```python
from build123d import *

# Parameters (mm, degrees)
F0_W      = 20
F0_H      = 20
F1_DEPTH  = 5
F2_W      = 1.8
F2_H      = 9.1
F2_H_2    = 1.8
F2_W_2    = 9.1
F3_DEPTH  = 2
F4_W      = 9
F4_H      = 1.7
F5_DEPTH  = 4
F6_W      = 9
F6_H      = 1.7
F7_DEPTH  = 4
F8_W      = 10
F8_H      = 2.2
F9_DEPTH  = 4
F10_W     = 10
F10_H     = 2.2
F11_DEPTH = 4
F12_W     = 2
F12_H     = 10
F13_DEPTH = 2.2
F14_W     = 10
F14_H     = 2
F15_DEPTH = 2.2
F16_W     = 9
F16_H     = 1.7
F17_DEPTH = 1.8
F18_W     = 1.7
F18_H     = 9
F19_DEPTH = 1.8


with BuildPart() as f1:
    # F0 (on Top) → F1 (new body)
    with BuildSketch(Plane.XY):
        with Locations((-15.7790486701, 11.8990262393)):
            Rectangle(F0_W, F0_H)
    extrude(amount=F1_DEPTH)

    # F2 (on face) → F3 (join)
    with BuildSketch(Plane.XY.offset(5)):
        with Locations((-15.7790486701, 17.3490262393)):
            Rectangle(F2_W, F2_H)
        with Locations((-15.7790486701, 11.8990262393)):
            Rectangle(F2_W, F2_H_2)
        with Locations((-21.2290486701, 11.8990262393)):
            Rectangle(F2_W_2, F2_H_2)
        with Locations((-10.3290486701, 11.8990262393)):
            Rectangle(F2_W_2, F2_H_2)
        with Locations((-15.7790486701, 6.4490262393)):
            Rectangle(F2_W, F2_H)
    extrude(amount=F3_DEPTH)

    # F4 (on face) → F5 (join)
    with BuildSketch(Plane.XZ.offset(-1.8990262393)):
        with Locations((-15.7790486701, 0.85)):
            Rectangle(F4_W, F4_H)
    extrude(amount=F5_DEPTH)

    # F6 (on face) → F7 (join)
    with BuildSketch(Plane(origin=(-25.7790486701, 0, 0), x_dir=(0, -1, 0), z_dir=(-1, 0, 0))):
        with Locations((-11.8990262393, 0.85)):
            Rectangle(F6_W, F6_H)
    extrude(amount=F7_DEPTH)

    # F8 (on face) → F9 (cut)
    with BuildSketch(Plane(origin=(0, 21.8990262393, 0), x_dir=(-1, 0, 0), z_dir=(0, 1, 0))):
        with Locations((15.7790486701, 1.1)):
            Rectangle(F8_W, F8_H)
    extrude(amount=-F9_DEPTH, mode=Mode.SUBTRACT)

    # F10 (on face) → F11 (cut)
    with BuildSketch(Plane.YZ.offset(-5.7790486701)):
        with Locations((11.8990262393, 1.1)):
            Rectangle(F10_W, F10_H)
    extrude(amount=-F11_DEPTH, mode=Mode.SUBTRACT)

    # F12 (on face) → F13 (cut)
    with BuildSketch(Plane(origin=(0, 0, 2.2), x_dir=(1, 0, 0), z_dir=(0, 0, -1))):
        with Locations((-8.7790486701, -11.8990262393)):
            Rectangle(F12_W, F12_H)
    extrude(amount=-F13_DEPTH, mode=Mode.SUBTRACT)

    # F14 (on face) → F15 (cut)
    with BuildSketch(Plane(origin=(0, 0, 2.2), x_dir=(1, 0, 0), z_dir=(0, 0, -1))):
        with Locations((-15.7790486701, -18.8990262393)):
            Rectangle(F14_W, F14_H)
    extrude(amount=-F15_DEPTH, mode=Mode.SUBTRACT)

    # F16 (on face) → F17 (join)
    with BuildSketch(Plane.XY.offset(1.7)):
        with Locations((-15.7790486701, -1.2509737607)):
            Rectangle(F16_W, F16_H)
    extrude(amount=F17_DEPTH)

    # F18 (on face) → F19 (join)
    with BuildSketch(Plane.XY.offset(1.7)):
        with Locations((-28.9290486701, 11.8990262393)):
            Rectangle(F18_W, F18_H)
    extrude(amount=F19_DEPTH)


solid = f1.part
```
Here's how the part is built. I have some questions about the finished solid (model axes, mm). A direction names the side the tool comes from. Coordinates: 2 decimals unless noted, no trailing zeros. Order: outer loops, then holes, each group sorted by start corner. A loop starts at its lowest first (then second) coordinate and runs counter-clockwise, first axis right, second up.
Item 1: Thinking about a two-plate mould opening in Y: for faces 1 (the face through (-5.779, 12, 3)), 2 (the face through (-16, 19, 4.4)), 3 (the face through (-28, 16.399, 1)), which applies, pulls with the +Y half, pulls with the -Y half, needs draft (parallel to the pull), parting line crosses it, or undercut?
Response values:
face 1: needs draft
face 2: undercut
face 3: pulls with the +Y half
Item 2: Which directions (+Z, -Z, +X, -X, +Y, -Y) give clear straight access to the entire face, cutting with the end or side of a thin tool? Please do faces 4 (the face through (-7.779, 12, 3)), 5 (the face through (-11.279, -1, 1)), 6 (the face through (-29, 12, 3.5)), 7 (the face through (-16, 1, 1.7)).
Response values:
face 4: -Z
face 5: +Z, -Z, +X, -Y
face 6: +Z, -X, +Y, -Y
face 7: +Z, +X, -X
Item 3: If we section it at A-A, the plane y = 5: List the corners of the cut face in (x, z) for me.
Response values:
outline: (-25.78, 0) - (-5.78, 0) - (-5.78, 5) - (-14.88, 5) - (-14.88, 7) - (-16.68, 7) - (-16.68, 5) - (-25.78, 5) - close
Item 4: If we section it at B-B, the plane z = 6.25: List the corners of the cut face in (x, y) for me.
Response values:
outline: (-25.78, 11) - (-16.68, 11) - (-16.68, 1.9) - (-14.88, 1.9) - (-14.88, 11) - (-5.78, 11) - (-5.78, 12.8) - (-14.88, 12.8) - (-14.88, 21.9) - (-16.68, 21.9) - (-16.68, 12.8) - (-25.78, 12.8) - close
Item 5: If we section it at C-C, the plane x = -17.25: List the corners of the cut face in (y, z) for me, then the cut area to 3 significant figures.
Response values:
outline: (-2.1, 0) - (17.9, 0) - (17.9, 4.4) - (19.9, 4.4) - (19.9, 2.2) - (21.9, 2.2) - (21.9, 5) - (12.8, 5) - (12.8, 7) - (11, 7) - (11, 5) - (1.9, 5) - (1.9, 1.7) - (-0.4, 1.7) - (-0.4, 3.5) - (-2.1, 3.5) - close
area: 100 mm2
Item 6: I'm going to push flat-ended pins straight in: pin 1 Ø0.6 at (x, y) = (-6.5, 11.5) entering from -Z; pin 2 Ø1.5 at (x, y) = (-25, 13) entering from +Z; pin 3 Ø3 at (x, z) = (-28.5, 1.5) entering from -Y; pin 4 Ø1 at (x, z) = (-11, 6) entering from +Y. Where does each tip first touch, or does it pass through?
Response values:
pin 1: stops at z = 2.2
pin 2: stops at z = 7
pin 3: stops at y = 7.4
pin 4: stops at y = 12.8
Item 7: If we section it at D-D, the plane z = 1: List the corners of the cut face in (x, y) for me, then the cut area to 3 significant figures.
Response values:
outline: (-29.78, 7.4) - (-25.78, 7.4) - (-25.78, 1.9) - (-20.28, 1.9) - (-20.28, -2.1) - (-11.28, -2.1) - (-11.28, 1.9) - (-5.78, 1.9) - (-5.78, 6.9) - (-9.78, 6.9) - (-9.78, 16.9) - (-5.78, 16.9) - (-5.78, 21.9) - (-10.78, 21.9) - (-10.78, 17.9) - (-20.78, 17.9) - (-20.78, 21.9) - (-25.78, 21.9) - (-25.78, 16.4) - (-29.78, 16.4) - close
area: 392 mm2
Item 8: I need wall thicknesses on probe 1 along Y at (x, z) = (-16.25, 2.5); probe 2 along Y at (x, z) = (-8.75, 2.5); probe 3 along Y at (x, z) = (-16.25, 4). Which ranges of each line are inside material? Lowest first, please.
Response values:
probe 1: y = -2.1 to -0.4, 1.9 to 17.9, 19.9 to 21.9
probe 2: y = 1.9 to 6.9, 16.9 to 21.9
probe 3: y = 1.9 to 17.9, 19.9 to 21.9
